```python
from build123d import *

# Parameters (mm, degrees)
SKETCH1_W               = 270.5
SKETCH1_H               = 150
BOSS_EXTRUDE1_DEPTH     = 15
BOSS_EXTRUDE5_DEPTH     = 150
CUT_EXTRUDE7_DEPTH      = 311.185801218
CUT_EXTRUDE7_DEPTH_BACK = 311.185801218
SKETCH5_R               = 5
CUT_EXTRUDE8_DEPTH      = 8
CUT_EXTRUDE9_DEPTH      = 180
CHAMFER1_SIZE           = 2
SKETCH16_W              = 15
SKETCH16_H              = 20
CUT_EXTRUDE10_DEPTH     = 10
FILLET2_R               = 1
FILLET3_R               = 3


with BuildPart() as part:
    # Sketch1 → Boss-Extrude1 (new body)
    with BuildSketch(Plane(origin=(0, 0, 0), x_dir=(1, 0, 0), z_dir=(0, 1, 0))):
        with Locations((135.25, 75)):
            Rectangle(SKETCH1_W, SKETCH1_H)
    extrude(amount=BOSS_EXTRUDE1_DEPTH)

    # Sketch12 → Boss-Extrude5 (add)
    with BuildSketch(Plane.XY.offset(-150)):
        with BuildLine():
            Line((270.5, 0), (270.5, -7.956989195))
            ThreePointArc((270.5, -7.956989195), (135.159339828, -7.060511664), (0, 0))
            Line((0, 0), (270.5, 0))
        make_face()
    extrude(amount=BOSS_EXTRUDE5_DEPTH)

    # Sketch5 → Cut-Extrude7 (cut, two sides: drawn at the far end of the back side and taken through both)
    with BuildSketch(Plane(origin=(0, 15, 0), x_dir=(1, 0, 0), z_dir=(0, 1, 0)).offset(-CUT_EXTRUDE7_DEPTH_BACK)):
        with Locations(Location((33, 45, 0), (0, 0, 270))):
            Circle(SKETCH5_R)
        with Locations(Location((40, 119, 0), (0, 0, 270))):
            Circle(SKETCH5_R)
        with Locations(Location((65, 119, 0), (0, 0, 270))):
            Circle(SKETCH5_R)
        with Locations(Location((73, 45, 0), (0, 0, 270))):
            Circle(SKETCH5_R)
    extrude(amount=CUT_EXTRUDE7_DEPTH + CUT_EXTRUDE7_DEPTH_BACK, mode=Mode.SUBTRACT)

    # Sketch13 → Cut-Extrude8 (cut)
    with BuildSketch(Plane(origin=(0, 15, 0), x_dir=(1, 0, 0), z_dir=(0, 1, 0))):
        Polygon((40, 109.185045424), (48.5, 114.092522712), (48.5, 123.907477288), (40, 128.814954576), (31.5, 123.907477288), (31.5, 114.092522712), align=None)
        Polygon((65, 109.185045424), (73.5, 114.092522712), (73.5, 123.907477288), (65, 128.814954576), (56.5, 123.907477288), (56.5, 114.092522712), align=None)
        Polygon((33, 35.185045424), (41.5, 40.092522712), (41.5, 49.907477288), (33, 54.814954576), (24.5, 49.907477288), (24.5, 40.092522712), align=None)
        Polygon((73, 35.185045424), (81.5, 40.092522712), (81.5, 49.907477288), (73, 54.814954576), (64.5, 49.907477288), (64.5, 40.092522712), align=None)
    extrude(amount=-CUT_EXTRUDE8_DEPTH, mode=Mode.SUBTRACT)

    # Sketch15 → Cut-Extrude9 (cut)
    with BuildSketch(Plane(origin=(270.5, 0, 0), x_dir=(0, 0, -1), z_dir=(1, 0, 0))):
        Polygon((20, 15), (130, 15), (130, 5), (140, 5), (140, 0), (10, 0), (10, 5), (20, 5), align=None)
    extrude(amount=-CUT_EXTRUDE9_DEPTH, mode=Mode.SUBTRACT)

    # Chamfer1
    chamfer1_edges = [part.edges().sort_by_distance(p)[0] for p in [
        (0, 7.5, -150),
        (270.5, 3.521505402, -150),
        (270.5, 3.521505402, 0),
        (0, 7.5, 0),
    ]]
    chamfer(chamfer1_edges, length=CHAMFER1_SIZE)

    # Sketch16 → Cut-Extrude10 (cut)
    with BuildSketch(Plane(origin=(0, 15, 0), x_dir=(1, 0, 0), z_dir=(0, 1, 0))):
        with Locations((17.5, 20)):
            Rectangle(SKETCH16_W, SKETCH16_H)
        with Locations((17.5, 130)):
            Rectangle(SKETCH16_W, SKETCH16_H)
    extrude(amount=-CUT_EXTRUDE10_DEPTH, mode=Mode.SUBTRACT)

    # Fillet2
    fillet2_edges = [part.edges().sort_by_distance(p)[0] for p in [
        (270.5, 15, -139),
        (270.5, 10, -130),
        (270.5, 5, -135),
        (270.5, 2.5, -140),
        (270.5, 0, -75),
        (270.5, 2.5, -10),
        (270.5, 5, -15),
        (270.5, 10, -20),
        (270.5, 15, -11),
        (135.25, 15, -150),
        (135.25, 15, 0),
        (0, 15, -75),
    ]]
    fillet(fillet2_edges, radius=FILLET2_R - 0.0001)  # a hair under: the kernel refuses the full size

    # Fillet3
    fillet3_edges = [part.edges().sort_by_distance(p)[0] for p in [
        (10, 15, -130),
        (10, 15, -20),
    ]]
    fillet(fillet3_edges, radius=FILLET3_R)


solid = part.part
```
Verification items for the finished model (mm, model axes). A direction names the side the tool comes from. Coordinates: 2 decimals unless noted, no trailing zeros. Write each loop counter-clockwise with the first axis right and the second up, starting at its lowest first coordinate (ties: lowest second). Pieces come first, ordered by that corner, then holes. Notation, with made-up numbers: (58.5, 18) - (110.5, 18) arc R22 cw to (110.5, 38) - close; hole circle Ø5 at (32.25, -1.75). An arc over 180 degrees is marked (long way). One line per question, with ' | ' between items. Start each with the question number.
1. Gauge pin test, flat ends, axial feed: P1, Ø12, axis at x = 19.5, z = -15.5, coming from the +Y side; P2, Ø5, axis at x = 68.5, z = -118, coming from the +Y side; P3, Ø6, axis at x = 40, z = -119, coming from the -Y side; P4, Ø7.5, axis at y = 8, z = -47, coming from the +X side. Record the tip position at first contact, or that the pin passes through.
2. Access from +Z, -Z, +X, -X, +Y, -Y to the whole of each face (thin tool, end or side, straight path). Record for faces 1 (the flat face through (181, 10, -130)), 2 (the flat face through (18, 10, -10)), 3 (the flat face through (181, 5, -15)).
3. Section check B-B (x = 143.5). Enter the section's corners in (y, z), plus the area to 3 significant figures.
4. Section check A-A (z = -45). Enter the section's corners in (x, y), plus the area to 3 significant figures.
5. Draft check along Y on faces 4 (the flat face through (56.5, 11, -119)), 5 (the flat face through (29, 7, -41)), 6 (the flat face through (181, 5, -135)). Enter one of: released by +Y, released by -Y, zero draft, split by the parting line, or undercut.
6. Section check D-D (x = 220.5). Enter the section's corners in (y, z).
7. Section check C-C (z = -64). Enter the section's corners in (x, y).
8. Material ranges on line 1 along X through (y, z) = (4, -119); line 2 along X through (y, z) = (3.75, -45); line 3 along Z through (x, y) = (73, 1), recorded low to high.
Computed values:
1) P1: y = 15 | P2: y = 7 | P3: through | P4: x = 90.5
2) face 1: +X, +Y | face 2: +Y | face 3: +X
3) outline: (-7.29, -150) - (14, -150) arc R1 ccw to (15, -149) - (15, -130) - (5, -130) - (5, -140) - (0, -140) - (0, -10) - (5, -10) - (5, -20) - (15, -20) - (15, -1) arc R1 ccw to (14, 0) - (-7.29, 0) - close | area: 1,590 mm²
4) outline: (0, 0) arc R2970.45 ccw to (28, -1.97) - (28, 7) - (24.5, 7) - (24.5, 15) - (1, 15) arc R1 ccw to (0, 14) - close; (38, -2.61) arc R2970.45 ccw to (68, -4.32) - (68, 7) - (64.5, 7) - (64.5, 15) - (41.5, 15) - (41.5, 7) - (38, 7) - close; (78, -4.83) arc R2970.45 ccw to (270.5, -7.96) - (270.5, -1) arc R1 ccw to (269.5, 0) - (90.5, 0) - (90.5, 15) - (81.5, 15) - (81.5, 7) - (78, 7) - close | area: 2,510 mm²
5) face 4: zero draft | face 5: released by +Y | face 6: undercut
6) outline: (-8.34, -150) - (14, -150) arc R1 ccw to (15, -149) - (15, -130) - (5, -130) - (5, -140) - (0, -140) - (0, -10) - (5, -10) - (5, -20) - (15, -20) - (15, -1) arc R1 ccw to (14, 0) - (-8.34, 0) - close
7) outline: (0, 0) arc R2970.45 ccw to (270.5, -7.96) - (270.5, -1) arc R1 ccw to (269.5, 0) - (90.5, 0) - (90.5, 15) - (1, 15) arc R1 ccw to (0, 14) - close
8) line 1: 0 to 35, 45 to 60, 70 to 90.5 | line 2: 0 to 28, 38 to 68, 78 to 90.5 | line 3: -150 to -50, -40 to 0
